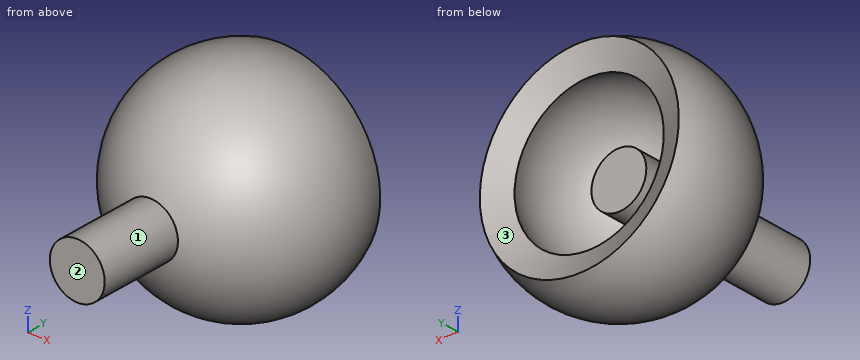
```python
from build123d import *

# Parameters (mm, degrees)
ESQUISSE2_R        = 2
BOSS_EXTRU_1_DEPTH = 14


with BuildPart() as part:
    # Esquisse1 → Révolution1 (revolve)
    with BuildSketch(Plane.XY, mode=Mode.PRIVATE) as r_volution1_sk:
        with BuildLine():
            Line((-7.250462296, 3.380946094), (-5.437846722, 2.53570957))
            ThreePointArc((-5.437846722, 2.53570957), (-5.060348675, -3.22379765), (0, -6))
            Line((0, -6), (0, -8))
            ThreePointArc((0, -8), (-6.747131567, -4.298396867), (-7.250462296, 3.380946094))
        make_face()
    revolve(r_volution1_sk.sketch.rotate(Axis((0, 0, 0), (0, -1, 0)), 270), axis=Axis((0, 0, 0), (0, -1, 0)))

    # Esquisse2 → Boss.-Extru.1 (add)
    with BuildSketch(Plane(origin=(0, 0, 0), x_dir=(1, 0, 0), z_dir=(0, 1, 0))):
        with Locations(Location((0, 0, 0), (0, 0, 270))):
            Circle(ESQUISSE2_R)
    extrude(amount=-BOSS_EXTRU_1_DEPTH)


solid = part.part
```
Read the model definition and answer for the solid it produces. Units are mm, in the model's axes. Face numbers are marked on the shaded views. Coordinates: 2 decimals unless noted, no trailing zeros. Order: outer loops, then holes, each group sorted by start corner. A loop starts at its lowest first (then second) coordinate and runs counter-clockwise, first axis right, second up. Notation, with made-up numbers: (88, 4.25) - (117, 4.25) arc R27 ccw to (117, 31.25) - close; hole circle Ø7 at (25.25, 14). An arc over 180 degrees is marked (long way). Answer as a JSON object with one key per item and string values. Group by question number.
Item 1: Flat-ended cylindrical pins translate along their axes: P1, Ø2, axis at x = 0, z = 1, coming from the +Y side; P2, Ø2, axis at x = 2.5, y = -2, coming from the +Z side; P3, Ø2, axis at x = 5.5, z = -2.5, coming from the +Y side. Find the tip coordinate at first contact, or state that the pin passes through.
Item 2: Section A-A (y = -4) is taken. Give the vertices of the cut face in (x, z), plus the area to 3 significant figures.
Item 3: Section D-D (y = -8.25) is taken. Give the vertices of the cut face in (x, z).
Item 4: Section B-B (z = 0) is taken. Give the vertices of the cut face in (x, y), plus the area to 3 significant figures.
Item 5: Consider probe 1 along X at (y, z) = (-2, 1.75); probe 2 along Y at (x, z) = (-1.5, 0); probe 3 along X at (y, z) = (-3, -0.25). Determine where each line is inside the solid, lowest interval first. Write a range as from..to.
Item 6: Section C-C (x = 0) is taken. Give the vertices of the cut face in (y, z), plus the area to 3 significant figures.
Item 7: The mould has two halves that part along Z. Classify the marked faces 1, 2 and 3: +Z half, -Z half, draft (parallel to the pull), parting line (faces both ways), or undercut.
Results are:
{
 "1": {"P1": "stops at y = 0", "P2": "stops at z = 7.69", "P3": "stops at y = 3.28"},
 "2": {"outline": "circle Ø13.86 at (0, 0); circle Ø4 at (0, 0); hole circle Ø8.94 at (0, 0)", "area": "101 mm^2"},
 "3": {"outline": "circle Ø4 at (0, 0)"},
 "4": {"outline": "(-7.25, 3.38) arc R8 ccw to (-2, -7.75) - (-2, -14) - (2, -14) - (2, -7.75) arc R8 ccw to (7.25, 3.38) - (5.44, 2.54) arc R6 cw to (2, -5.66) - (2, 0) - (-2, 0) - (-2, -5.66) arc R6 cw to (-5.44, 2.54) - close", "area": "104 mm^2"},
 "5": {"probe 1": "x = -7.55..-5.38, -0.97..0.97, 5.38..7.55", "probe 2": "y = -14..0", "probe 3": "x = -7.41..-5.19, -1.98..1.98, 5.19..7.41"},
 "6": {"outline": "(-14, -2) - (-7.75, -2) arc R8 ccw to (3.38, -7.25) - (2.54, -5.44) arc R6 cw to (-5.66, -2) - (0, -2) - (0, 2) - (-5.66, 2) arc R6 cw to (2.54, 5.44) - (3.38, 7.25) arc R8 ccw to (-7.75, 2) - (-14, 2) - close", "area": "104 mm^2"},
 "7": {"face 1": "parting line", "face 2": "draft", "face 3": "undercut"}
}
